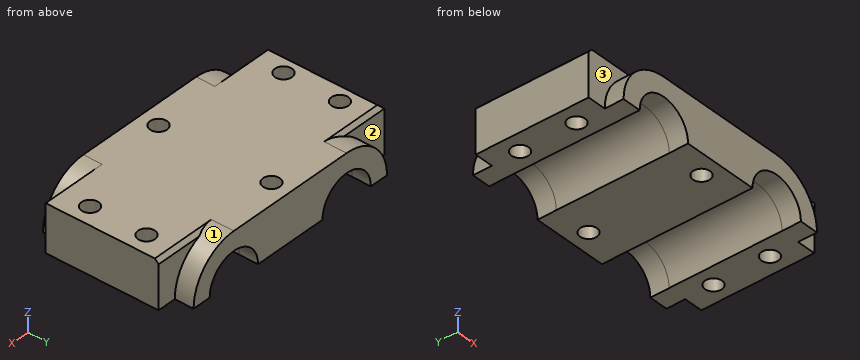
```python
from build123d import *

# Parameters (mm, degrees)
PAD_DEPTH         = 12.5
CHAMFER_SIZE      = 1
PAD001_DEPTH      = 5
PAD001_DEPTH_BACK = 35
SKETCH002_R       = 7.5
POCKET_DEPTH      = 35.001
SKETCH003_R       = 2.25
POCKET001_DEPTH   = 12.501


with BuildPart() as part:
    # Sketch → Pad (new body)
    with BuildSketch(Plane.XY):
        Polygon((-35, 15), (-35, -15), (-30, -15), (30, -15), (35, -15), (35, 15), (30, 15), (-30, 15), align=None)
    extrude(amount=PAD_DEPTH)

    # Chamfer
    chamfer_edges = [part.edges().sort_by_distance(p)[0] for p in [
        (0, 15, 12.5),
        (-35, 0, 12.5),
    ]]
    chamfer(chamfer_edges, length=CHAMFER_SIZE)

    # Sketch001 → Pad001 (new body, two sides)
    with BuildSketch(Plane.XZ.offset(15)) as pad001_sk:
        with BuildLine():
            ThreePointArc((-10, 0), (-17.5, 7.5), (-25, 0))
            Line((-25, 0), (-30, 0))
            ThreePointArc((-17.499993, 12.5), (-26.338832, 8.838837), (-30, 0))
            Line((-17.499993, 12.5), (17.500032, 12.5))
            ThreePointArc((30, 0), (26.338846, 8.838823), (17.500032, 12.5))
            Line((25, 0), (30, 0))
            ThreePointArc((25, 0), (17.5, 7.5), (10, 0))
            Line((10, 0), (-10, 0))
        make_face()
    extrude(amount=PAD001_DEPTH)
    extrude(pad001_sk.sketch, amount=-PAD001_DEPTH_BACK)

    # Sketch002 → Pocket (cut, through all)
    with BuildSketch(Plane(origin=(0, 15, 0), x_dir=(-1, 0, 0), z_dir=(0, 1, 0))):
        with Locations((-17.5, 0)):
            Circle(SKETCH002_R)
        with Locations((17.5, 0)):
            Circle(SKETCH002_R)
    extrude(amount=-POCKET_DEPTH, mode=Mode.SUBTRACT)

    # Sketch003 → Pocket001 (cut, through all)
    with BuildSketch(Plane.XY.offset(12.5)):
        with Locations((0, 15)):
            Circle(SKETCH003_R)
        with Locations((0, -15)):
            Circle(SKETCH003_R)
        with Locations((-30, 7.5)):
            Circle(SKETCH003_R)
        with Locations((-30, -7.5)):
            Circle(SKETCH003_R)
        with Locations((30, 7.5)):
            Circle(SKETCH003_R)
        with Locations((30, -7.5)):
            Circle(SKETCH003_R)
    extrude(amount=-POCKET001_DEPTH, mode=Mode.SUBTRACT)


solid = part.part
```
Work out the finished part from the listing and answer in its coordinate system (mm). Face numbers are marked on the shaded views. A direction names the side the tool comes from. Give positions to 0.01 mm unless a question says otherwise; leave off trailing zeros. Loops run counter-clockwise (first coordinate to the right, second up) from the corner with the lowest first, then second, coordinate; pieces in that order, holes last. Notation, with made-up numbers: M 27.5,-1 L 75.5,-1 A26 cw 75.5,24 Z; hole C 89.25,19.5 d9. An arc over 180 degrees is marked long. One line per item, written item: value. Start each with the question number.
1. Which of the six approach directions +Z, -Z, +X, -X, +Y, -Y give full straight-line access (tool end or side, diameter ignored) to the marked faces 1, 2 and 3?
2. Find section D-D (y = -2.5). Give the vertices of the cut face in (x, z).
3. Find section A-A (z = 3.5). State how many separate pieces and enclosed holes the cut face has, and give its area (3 significant figures).
4. Find section B-B (y = 7.5). Give the vertices of the cut face in (x, z).
5. Find section C-C (x = 0). Give the vertices of the cut face in (y, z), and give its area (4 significant figures).
6. Each of these flat-tipped pins is pushed along its axis until it touches: P1, Ø12, axis at x = -24.5, y = 10, coming from the -Z side; P2, Ø4, axis at x = 30.5, z = 7.5, coming from the -Y side. Where does it stop, or does it pass through?
7. Find the intervals of material crossed by probe 1 along Y at (x, z) = (-30, 4.25); probe 2 along Y at (x, z) = (0, 9.5); probe 3 along X at (y, z) = (-16.5, 1.5), in increasing order.
Reported:
1. face 1: +Z, +X, +Y
1. face 2: +Z, -X, +Y
1. face 3: +Z, -X, -Y
2. outline: M -35,0 L -25,0 A7.5 cw -10,0 L 10,0 A7.5 cw 25,0 L 35,0 L 35,12.5 L -34,12.5 L -35,11.5 Z
3. separate pieces: 3
3. enclosed holes: 6
3. area: 1,530 mm²
4. outline: M -35,0 L -32.25,0 L -32.25,12.5 L -34,12.5 L -35,11.5 Z; M -27.75,0 L -25,0 A7.5 cw -10,0 L 10,0 A7.5 cw 25,0 L 27.75,0 L 27.75,12.5 L -27.75,12.5 Z; M 32.25,0 L 35,0 L 35,12.5 L 32.25,12.5 Z
5. outline: M -20,0 L -17.25,0 L -17.25,12.5 L -20,12.5 Z; M -12.75,0 L 12.75,0 L 12.75,12.5 L -12.75,12.5 Z; M 17.25,0 L 20,0 L 20,12.5 L 17.25,12.5 Z
5. area: 387.5 mm²
6. P1: stops at z = 0
6. P2: stops at y = -15
7. probe 1: y = -15 to -9.75, -5.25 to 5.25, 9.75 to 15
7. probe 2: y = -20 to -17.25, -12.75 to 12.75, 17.25 to 20
7. probe 3: x = -29.91 to -24.85, -10.15 to -1.68, 1.68 to 10.15, 24.85 to 29.91
